Verification items for the finished model (mm, model axes). A direction names the side the tool comes from. Give positions to 0.01 mm unless a question says otherwise; leave off trailing zeros. Loops run counter-clockwise (first coordinate to the right, second up) from the corner with the lowest first, then second, coordinate; pieces in that order, holes last. Notation, with made-up numbers: (85.5, 35.5) - (105.5, 35.5) arc R31 cw to (105.5, 73.5) - close; hole circle Ø3 at (51.5, 46). An arc over 180 degrees is marked (long way). One line per question, with ' | ' between items. Start each with the question number.
1. Section check D-D, the plane x = 141.5. Enter the section's corners in (y, z).
2. Thickness scan on line 1 along X through (y, z) = (-61.5, -3); line 2 along Z through (x, y) = (-9, -16); line 3 along X through (y, z) = (-141.5, -31). Record the ranges inside material, lowest first. Write a range as from..to.
3. Depth check by flat-ended pin: pin 1 Ø3 at (y, z) = (-108, -15.5) entering from -X; pin 2 Ø21 at (x, z) = (-6.5, -18) entering from +Y; pin 3 Ø12 at (x, z) = (-13, -33.5) entering from -Y. Enter the tip coordinate at first touch or a pass-through.
4. Mould release check, pull along X, two halves, no side actions. Record for faces 1 (the face through (0, -132, -70)), 2 (the face through (-3, 3, 0)), 3 (the face through (-100, -56, -35)): +X half, -X half, draft (parallel to the pull), parting line (faces both ways), or undercut.
5. Section check B-B, the plane y = -145. Enter the section's corners in (x, z), then the cut area to 3 significant figures.
6. Section check A-A, the plane x = -19.5. Enter the section's corners in (y, z).
7. Section check C-C, the plane y = -35.5. Enter the section's corners in (x, z).
8. Tool access check on faces 4 (the face through (100, -56, -35)), 5 (the face through (81, -45, -35)), 6 (the face through (-1, -150, -35)), 7 (the face through (-90.633, 38.416, -34.51)). Record the directions out of +Z, -Z, +X, -X, +Y, -Y that give a thin tool (end or side, any length) a straight path to the whole face; none if there is none.
from build123d import *

# Parameters (mm, degrees)
SKETCH1_W           = 360
SKETCH1_H           = 360
BOSS_EXTRUDE1_DEPTH = 6
SKETCH2_W           = 200
SKETCH2_H           = 19
BOSS_EXTRUDE2_DEPTH = 70
BOSS_EXTRUDE3_DEPTH = 19


with BuildPart() as part:
    # Sketch1 → Boss-Extrude1 (new body)
    with BuildSketch(Plane.XY):
        Rectangle(SKETCH1_W, SKETCH1_H)
    extrude(amount=BOSS_EXTRUDE1_DEPTH)

    # Sketch2 → Boss-Extrude2 (add)
    with BuildSketch(Plane.XY):
        with Locations((0, -140.5)):
            Rectangle(SKETCH2_W, SKETCH2_H)
    extrude(amount=-BOSS_EXTRUDE2_DEPTH)

    # Sketch3 → Boss-Extrude3 (add)
    with BuildSketch(Plane(origin=(100, 0, 0), x_dir=(0, 0, -1), z_dir=(1, 0, 0))):
        Polygon((0, -131), (0, 86.467943448), (70, -11), (70, -131), align=None)
    boss_extrude3 = extrude(amount=-BOSS_EXTRUDE3_DEPTH)

    # Mirror1: Boss-Extrude3 across plane
    add(boss_extrude3.mirror(Plane(origin=(0, 0, 0), x_dir=(0, 0, 1), z_dir=(1, 0, 0))))


solid = part.part
Results list:
1) outline: (-180, 0) - (180, 0) - (180, 6) - (-180, 6) - close
2) line 1: -100..-81, 81..100 | line 2: 0..6 | line 3: -100..100
3) pin 1: x = -100 | pin 2: y = -131 | pin 3: y = -150
4) face 1: draft | face 2: undercut | face 3: -X half
5) outline: (-180, 0) - (-100, 0) - (-100, -70) - (100, -70) - (100, 0) - (180, 0) - (180, 6) - (-180, 6) - close | area: 16,200 mm²
6) outline: (-180, 0) - (-150, 0) - (-150, -70) - (-131, -70) - (-131, 0) - (180, 0) - (180, 6) - (-180, 6) - close
7) outline: (-180, 0) - (-100, 0) - (-100, -70) - (-81, -70) - (-81, 0) - (81, 0) - (81, -70) - (100, -70) - (100, 0) - (180, 0) - (180, 6) - (-180, 6) - close
8) face 4: -Z, +X, +Y, -Y | face 5: -Z, +Y | face 6: -Z, +X, -X, -Y | face 7: -Z, +X, -X, +Y
